The listing builds one solid part. Answer for the finished solid, in the listing's coordinates (mm). Face numbers are marked on the shaded views. A direction names the side the tool comes from. Coordinates: 2 decimals unless noted, no trailing zeros. Order: outer loops, then holes, each group sorted by start corner. A loop starts at its lowest first (then second) coordinate and runs counter-clockwise, first axis right, second up. Notation, with made-up numbers: (89, -27) -> (115, -27) arc R19 ccw to (115, -23) -> close; hole circle Ø9 at (-20, 85). An arc over 180 degrees is marked (long way). Return JSON: item names as keys, results as strings.
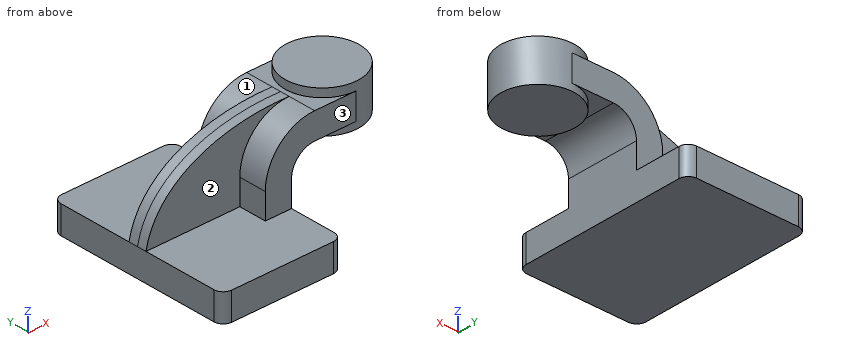
from build123d import *

# Parameters (mm, degrees)
F1_DEPTH = 63.5
F0_W     = 25.4
F0_H     = 18.034
F2_DEPTH = 25.4
F3_DEPTH = 6.35
F5_R     = 6.35


with BuildPart() as f1:
    # F0 (on Front) → F1 (new body, symmetric)
    with BuildSketch(Plane.XZ):
        Polygon((-41.275, 9.525), (-41.275, -9.525), (41.275, -9.525), (41.275, 9.525), (23.241, 9.525), align=None)
    extrude(amount=F1_DEPTH, both=True)

    # F0 (on Front) → F2 (join, symmetric)
    with BuildSketch(Plane.XZ):
        with BuildLine():
            Line((23.241, 9.525), (41.275, 9.525))
            Line((41.275, 9.525), (41.275, 27.0002))
            ThreePointArc((41.275, 27.0002), (45.9246798487, 38.2255201513), (57.15, 42.8752))
            Line((57.15, 42.8752), (60.325, 42.8752))
            Line((60.325, 42.8752), (60.325, 60.9092))
            Line((60.325, 60.9092), (57.15, 60.9092))
            ThreePointArc((57.15, 60.9092), (33.1727161567, 50.9774838433), (23.241, 27.0002))
            Line((23.241, 27.0002), (23.241, 9.525))
        make_face()
        with Locations((73.025, 51.8922)):
            Rectangle(F0_W, F0_H)
    extrude(amount=F2_DEPTH, both=True)

    # F0 (on Front) → F3 (join, symmetric)
    with BuildSketch(Plane.XZ):
        with BuildLine():
            add(Edge.make_bspline(
                [(-41.275, 9.525), (-34.2406501154, 46.4476686137), (10.1438477317, 62.8272760307), (57.15, 60.9092)],
                knots=[0, 0, 0, 0, 111.0307013156, 111.0307013156, 111.0307013156, 111.0307013156], degree=3))
            Line((-41.275, 9.525), (23.241, 9.525))
            Line((23.241, 9.525), (23.241, 27.0002))
            ThreePointArc((23.241, 27.0002), (33.1727161567, 50.9774838433), (57.15, 60.9092))
        make_face()
    extrude(amount=F3_DEPTH, both=True)

    # F0 (on Front) → F4 (revolve)
    with BuildSketch(Plane.XZ):
        Polygon((85.725, 66.675), (85.725, 60.9092), (85.725, 42.8752), (85.725, 38.1), (111.125, 38.1), (111.125, 66.675), align=None)
    revolve(axis=Axis((85.725, 0, 52.3875), (0, 0, -1)))

    # F5
    f5_edges = [f1.edges().sort_by_distance(p)[0] for p in [
        (-41.275, -63.5, 0),
        (41.275, -63.5, 0),
        (-41.275, 63.5, 0),
        (41.275, 63.5, 0),
    ]]
    fillet(f5_edges, radius=F5_R)


solid = f1.part
1. The part is cut by section C-C on y = -51. Give the vertices of the cut face in (x, z) (3 decimals).
Answer block:
{"outline": "(-41.275, -9.525) -> (41.275, -9.525) -> (41.275, 9.525) -> (-41.275, 9.525) -> close"}
2. The part is cut by section A-A on y = -18. Give the vertices of the cut face in (x, z) (3 decimals).
Answer block:
{"outline": "(-41.275, -9.525) -> (41.275, -9.525) -> (41.275, 27) arc R15.875 cw to (57.15, 42.875) -> (67.804, 42.875) -> (67.804, 38.1) -> (103.646, 38.1) -> (103.646, 66.675) -> (67.804, 66.675) -> (67.804, 60.909) -> (57.15, 60.909) arc R33.909 ccw to (23.241, 27) -> (23.241, 9.525) -> (-41.275, 9.525) -> close"}
3. Consider line 1 (Z direction, x = 27, y = 44) (3 decimals); line 2 (X direction, y = 18, z = 4) (3 decimals); line 3 (Z direction, x = 65, y = -8) (3 decimals). Determine where each line is inside the solid, lowest interval first. Write a range as from..to.
Answer block:
{"line 1": "z = -9.525..9.525", "line 2": "x = -41.275..41.275", "line 3": "z = 38.1..66.675"}
4. The part is cut by section B-B on y = 14. Give the vertices of the cut face in (x, z) (3 decimals), and give its area (3 significant figures).
Answer block:
{"outline": "(-41.275, -9.525) -> (41.275, -9.525) -> (41.275, 27) arc R15.875 cw to (57.15, 42.875) -> (64.532, 42.875) -> (64.532, 38.1) -> (106.918, 38.1) -> (106.918, 66.675) -> (64.532, 66.675) -> (64.532, 60.909) -> (57.15, 60.909) arc R33.909 ccw to (23.241, 27) -> (23.241, 9.525) -> (-41.275, 9.525) -> close", "area": "3,940 mm2"}
5. Each of these flat-tipped pins is pushed along its axis until it touches: pin 1 Ø12 at (y, z) = (-14.5, 26) entering from +X; pin 2 Ø14 at (y, z) = (-16.5, 19.5) entering from -X; pin 3 Ø8.5 at (x, y) = (74, 9.5) entering from -Z. Where does it stop, or does it pass through?
Answer block:
{"pin 1": "stops at x = 42.08", "pin 2": "stops at x = 23.24", "pin 3": "stops at z = 38.1"}
6. For the marked faces 1, 2 and 3, determine the directions among +Z, -Z, +X, -X, +Y, -Y from which every point of the face is accessible in a straight line to the end or side of a thin tool.
Answer block:
{"face 1": "+Z, -X, +Y", "face 2": "+Z, -X, -Y", "face 3": "+Z, +X, -X, -Y"}
